Work out the finished part from the listing and answer in its coordinate system (mm). A direction names the side the tool comes from. Give positions to 0.01 mm unless a question says otherwise; leave off trailing zeros. Loops run counter-clockwise (first coordinate to the right, second up) from the corner with the lowest first, then second, coordinate; pieces in that order, holes last.
Autodesk Inventor part; units mm, degrees
ref_plane "YZ Plane" through (0, 0, 0) normal (1, 0, 0) x (0, 1, 0)
ref_plane "XZ Plane" through (0, 0, 0) normal (0, 1, 0) x (-1, 0, 0)
ref_plane "XY Plane" through (0, 0, 0) normal (0, 0, 1) x (1, 0, 0)
sketch "Sketch1" plane through (0, 0, 0) normal (0, 0, 1) x (1, 0, 0)
  line L0 (-37.5, -35) -> (37.5, -35)
  line L1 (37.5, -35) -> (37.5, 35)
  line L2 (37.5, 35) -> (-37.5, 35)
  line L3 (-37.5, 35) -> (-37.5, -35)
  line L4 (-37.5, -35) -> (37.5, 35) construction
  line L5 (37.5, -35) -> (-37.5, 35) construction
  point P0 (0, 0)
  dimension "d0" = 75
  dimension "d1" = 70
extrude "Extrusion1" add sketch "Sketch1" along normal blind 5
sketch "Sketch2" plane through (0, 0, 5) normal (0, 0, 1) x (1, 0, 0)
  line L0 (-30, -30) -> (30, -30) construction
  line L1 (-37.5, -35) -> (37.5, -35) construction
  line L2 (-30, 23) -> (30, 23) construction
  point P0 (0, 0)
  point P1 (0, -30)
  dimension "d4" = 60
  dimension "d5" = 5
  dimension "d6" = 60
  dimension "d7" = 58
  dimension "d8" = 30
hole "Hole1" at (-30, -30, 5) at (30, -30, 5) at (30, 23, 5) at (-30, 23, 5) direction (0, 0, -1) diameter 5.5 depth 8 tip angle 118
fillet "Fillet1" radius 4 4 edges at (-37.5, 35, 2.5) (37.5, 35, 2.5) (-37.5, -35, 2.5) (37.5, -35, 2.5)
sketch "Sketch3" plane through (0, 0, 5) normal (0, 0, 1) x (1, 0, 0)
  circle A0 centre (30, 23) radius 2.75
  line L0 (27.25, 23) -> (27.25, 35)
  line L1 (33.5, 35) -> (-33.5, 35)
  line L2 (32.75, 23) -> (32.75, 35)
  line L3 (32.75, 35) -> (27.25, 35)
  line L4 (32.75, 23) -> (27.25, 23)
  point P0 (0, 0)
extrude "Extrusion2" cut sketch "Sketch3" against normal blind 5 contours A0 L0 L1 L2
properties part number "Halter_Tesla" material "Polycarbonate, Clear"
Item 1: Find section B-B, the plane x = -30. Write down the section's boundary in (y, z).
Item 2: For faces 1 (the face through (32.75, 29, 3)), 2 (the face through (0, -35, 2)), determine the directions among +Z, -Z, +X, -X, +Y, -Y from which every point of the face is accessible in a straight line to the end or side of a thin tool.
Item 3: Find section C-C, the plane z = 2.85. Write down the section's boundary in (x, y), plus the area to 3 significant figures.
Item 4: Find section D-D, the plane x = 30. Write down the section's boundary in (y, z).
Item 5: A flat-ended cylindrical pin translates along its axis: pin 1 Ø7 at (x, y) = (-30, -30) entering from +Z. Find the tip coordinate at first contact, or state that the pin passes through.
Item 6: Find section A-A, the plane y = -30. Write down the section's boundary in (x, z), plus the area to 3 significant figures.
Item 7: Consider line 1 (X direction, y = -30, z = 3.15); line 2 (Y direction, x = -30, z = 1); line 3 (Y direction, x = 30, z = 1). Determine where each line is inside the solid, lowest interval first.
Item 8: Determine the mould class of faces 3 (the face through (-36.297, 33.859, 2.535)), 4 (the face through (-1, 0, 0)), 5 (the face through (-31.859, -27.973, 2.465)) for opening direction X: released by +X, released by -X, zero draft, split by the parting line, or undercut.
Ans:
1. outline: (-35, 0) - (-32.75, 0) - (-32.75, 5) - (-35, 5) - close; (-27.25, 0) - (20.25, 0) - (20.25, 5) - (-27.25, 5) - close; (25.75, 0) - (35, 0) - (35, 5) - (25.75, 5) - close
2. face 1: +Z, -Z, +Y
2. face 2: +Z, -Z, +X, -X, -Y
3. outline: (-37.5, -31) arc R4 ccw to (-33.5, -35) - (33.5, -35) arc R4 ccw to (37.5, -31) - (37.5, 31) arc R4 ccw to (33.5, 35) - (32.75, 35) - (32.75, 23) arc R2.75 cw to (27.25, 23) - (27.25, 35) - (-33.5, 35) arc R4 ccw to (-37.5, 31) - close; hole circle Ø5.5 at (-30, -30); hole circle Ø5.5 at (-30, 23); hole circle Ø5.5 at (30, -30)
3. area: 5,090 mm2
4. outline: (-35, 0) - (-32.75, 0) - (-32.75, 5) - (-35, 5) - close; (-27.25, 0) - (20.25, 0) - (20.25, 5) - (-27.25, 5) - close
5. pin 1: stops at z = 5
6. outline: (-37.5, 0) - (-32.75, 0) - (-32.75, 5) - (-37.5, 5) - close; (-27.25, 0) - (27.25, 0) - (27.25, 5) - (-27.25, 5) - close; (32.75, 0) - (37.5, 0) - (37.5, 5) - (32.75, 5) - close
6. area: 320 mm2
7. line 1: x = -37.5 to -32.75, -27.25 to 27.25, 32.75 to 37.5
7. line 2: y = -35 to -32.75, -27.25 to 20.25, 25.75 to 35
7. line 3: y = -35 to -32.75, -27.25 to 20.25
8. face 3: released by -X
8. face 4: zero draft
8. face 5: undercut
